```python
from build123d import *

# Parameters (mm, degrees)
SKETCH_1_R          = 5.05
SKETCH_1_R_2        = 13
EXTRUDE_1_DEPTH     = 12
FILLET_1_R          = 3
CUT_EXTRUDE_3_DEPTH = 277.39464539
FILLET_2_R          = 3
EXTRUDE_START       = -12
SKETCH_5_R          = 40
SKETCH_5_R_2        = 5.05
EXTRUDE_2_DEPTH     = 12
FILLET_3_R          = 6
EXTRUDE_3_DEPTH     = 12
FILLET_4_R          = 3
SKETCH_8_R          = 32
CUT_EXTRUDE_5_DEPTH = 279.152835686


with BuildPart() as part:
    # 草图1 → 凸台-拉伸1 (new body)
    with BuildSketch(Plane(origin=(0, 0, 0), x_dir=(1, 0, 0), z_dir=(0, 1, 0))):
        with BuildLine():
            Line((-17.992942616, -0.504), (-24.990198078, 249.3))
            ThreePointArc((-24.990198078, 249.3), (0, 275), (24.990198078, 249.3))
            Line((24.990198078, 249.3), (17.992942616, -0.504))
            ThreePointArc((17.992942616, -0.504), (0, -18), (-17.992942616, -0.504))
        make_face()
        with Locations(Location((0, 0, 0), (0, 0, 270))):
            Circle(SKETCH_1_R, mode=Mode.SUBTRACT)
        with Locations(Location((0, 250, 0), (0, 0, 270))):
            Circle(SKETCH_1_R_2, mode=Mode.SUBTRACT)
        Polygon((-16.444447487, 158.5), (-17.704941698, 203.5), (11.028871219, 137.174942267), align=None, mode=Mode.SUBTRACT)
        Polygon((15.954255294, 141), (18.475243716, 231), (-12, 219.5), align=None, mode=Mode.SUBTRACT)
    extrude(amount=EXTRUDE_1_DEPTH)

    # 圆角1
    fillet_1_edges = [part.edges().sort_by_distance(p)[0] for p in [
        (-16.444447487, 6, -158.5),
        (11.028871219, 6, -137.174942267),
        (-17.704941698, 6, -203.5),
        (18.475243716, 6, -231),
        (-12, 6, -219.5),
        (15.954255294, 6, -141),
    ]]
    fillet(fillet_1_edges, radius=FILLET_1_R)

    # 草图4 → 切除-拉伸3 (cut, through all)
    with BuildSketch(Plane(origin=(0, 12, 0), x_dir=(1, 0, 0), z_dir=(0, 1, 0))):
        Polygon((-13.050343026, 144.472367448), (12.494927596, 124.643879429), (9.742058902, 26.365688077), (-10.175105816, 41.825585442), align=None)
    extrude(amount=-CUT_EXTRUDE_3_DEPTH, mode=Mode.SUBTRACT)

    # 圆角2
    fillet_2_edges = [part.edges().sort_by_distance(p)[0] for p in [
        (-10.175105816, 6, -41.825585442),
        (-13.050343026, 6, -144.472367448),
        (9.742058902, 6, -26.365688077),
    ]]
    fillet(fillet_2_edges, radius=FILLET_2_R)

    # 草图5 → 凸台-拉伸2 (add)
    with BuildSketch(Plane(origin=(0, 12, 0), x_dir=(1, 0, 0), z_dir=(0, 1, 0)).offset(EXTRUDE_START)):
        Circle(SKETCH_5_R)
        with Locations(Location((0, 0, 0), (0, 0, 270))):
            Circle(SKETCH_5_R_2, mode=Mode.SUBTRACT)
    extrude(amount=EXTRUDE_2_DEPTH)

    # 圆角3
    fillet_3_edges = [part.edges().sort_by_distance(p)[0] for p in [
        (18.993134598, 6, -35.203136766),
        (-18.993134598, 6, -35.203136766),
    ]]
    fillet(fillet_3_edges, radius=FILLET_3_R)

    # 草图6 → 凸台-拉伸3 (add)
    with BuildSketch(Plane(origin=(0, 12, 0), x_dir=(1, 0, 0), z_dir=(0, 1, 0))):
        Polygon((9.60137553, 125.435937788), (-13.068657882, 42.617643801), (-7.609801347, 39.834371112), (-7.28155375, 41.033527083), (15.388479662, 123.85182107), (9.929623127, 126.635093759), align=None)
    extrude(amount=-EXTRUDE_3_DEPTH)

    # 圆角4
    # the kernel refuses this fillet: 3 mm, written as the material it adds along each edge
    with BuildSketch(Plane(origin=(12.14036175, 0, -111.985778385), x_dir=(-0.028000000000000382, 0, 0.9996079231378672), z_dir=(0, 1, 0))) as fillet_4_piece_1:
        with BuildLine():
            CenterArc((FILLET_4_R * 8.32187878655, -FILLET_4_R), FILLET_4_R, 90, 166.295794849)
            Line((FILLET_4_R * 8.08496933551, -FILLET_4_R * 1.97153173495), (FILLET_4_R * 8.08023114649, -FILLET_4_R * 1.99096236965))
            Line((FILLET_4_R * 8.08023114649, -FILLET_4_R * 1.99096236965), (-FILLET_4_R * 0.0047381890208, -FILLET_4_R * 0.0194306346989))
            Line((-FILLET_4_R * 0.0047381890208, -FILLET_4_R * 0.0194306346989), (0, FILLET_4_R * 0.02))
            Line((0, FILLET_4_R * 0.02), (FILLET_4_R * 8.32187878655, FILLET_4_R * 0.02))
            Line((FILLET_4_R * 8.32187878655, FILLET_4_R * 0.02), (FILLET_4_R * 8.32187878655, 0))
        make_face()
    extrude(amount=12)
    with BuildSketch(Plane(origin=(-10.463842583, 0, -52.133569747), x_dir=(-0.02799999999999904, 0, -0.9996079231378672), z_dir=(0, 1, 0))) as fillet_4_piece_2:
        with BuildLine():
            CenterArc((FILLET_4_R * 6.72600834912, -FILLET_4_R), FILLET_4_R, 90, 163.086811796)
            Line((FILLET_4_R * 6.43508592619, -FILLET_4_R * 1.95674664558), (FILLET_4_R * 6.42926747773, -FILLET_4_R * 1.9758815785))
            Line((FILLET_4_R * 6.42926747773, -FILLET_4_R * 1.9758815785), (-FILLET_4_R * 0.00581844845863, -FILLET_4_R * 0.0191349329117))
            Line((-FILLET_4_R * 0.00581844845863, -FILLET_4_R * 0.0191349329117), (0, FILLET_4_R * 0.02))
            Line((0, FILLET_4_R * 0.02), (FILLET_4_R * 6.72600834912, FILLET_4_R * 0.02))
            Line((FILLET_4_R * 6.72600834912, FILLET_4_R * 0.02), (FILLET_4_R * 6.72600834912, 0))
        make_face()
    extrude(amount=12)
    with BuildSketch(Plane(origin=(9.929623127, 12, -126.635093759), x_dir=(-0.7899521186549702, 0, -0.6131685333026506), z_dir=(0, -1, 0))) as fillet_4_piece_3:
        with BuildLine():
            CenterArc((FILLET_4_R * 0.668049057951, -FILLET_4_R), FILLET_4_R, 90, 67.489733811)
            Line((-FILLET_4_R * 0.255761890972, -FILLET_4_R * 0.617151034153), (-FILLET_4_R * 0.27423810995, -FILLET_4_R * 0.609494054836))
            Line((-FILLET_4_R * 0.27423810995, -FILLET_4_R * 0.609494054836), (-FILLET_4_R * 0.013360981159, FILLET_4_R * 0.02))
            Line((-FILLET_4_R * 0.013360981159, FILLET_4_R * 0.02), (FILLET_4_R * 0.668049057951, FILLET_4_R * 0.02))
            Line((FILLET_4_R * 0.668049057951, FILLET_4_R * 0.02), (FILLET_4_R * 0.668049057951, 0))
        make_face()
    extrude(amount=12)
    with BuildSketch(Plane(origin=(-7.609801347, 12, -39.834371112), x_dir=(0.789952118654971, 0, 0.6131685333026496), z_dir=(0, -1, 0))) as fillet_4_piece_4:
        with BuildLine():
            CenterArc((2.149138752, -2.650136686), FILLET_4_R, 117.947316923, 39.542416888)
            Line((-0.622294094, -1.501589789), (-0.677722751, -1.478618851))
            Line((-0.677722751, -1.478618851), (-0.055428657, 0.022970938))
            Line((-0.055428657, 0.022970938), (0, 0.06))
            ThreePointArc((0, 0.06), (0.371580126, 0.06), (0.715040682, 0.053002734))
            Line((0.715040682, 0.053002734), (0.743160252, 0))
        make_face()
    extrude(amount=12)

    # 草图8 → 切除-拉伸5 (cut, through all)
    with BuildSketch(Plane(origin=(0, 12, 0), x_dir=(1, 0, 0), z_dir=(0, 1, 0))):
        with Locations(Location((0, 0, 0), (0, 0, 270))):
            Circle(SKETCH_8_R)
    extrude(amount=-CUT_EXTRUDE_5_DEPTH, mode=Mode.SUBTRACT)


solid = part.part
```
Can you work these out from the model? Positions are in its coordinate system, mm. A direction names the side the tool comes from. Coordinates: 2 decimals unless noted, no trailing zeros. Loops run counter-clockwise (first coordinate to the right, second up) from the corner with the lowest first, then second, coordinate; pieces in that order, holes last. Notation, with made-up numbers: (67, 24) -> (120, 24) arc R21 ccw to (120, 60) -> close; hole circle Ø3 at (31.25, 44). An arc over 180 degrees is marked (long way). Put each result on its own line as item: value. Start each with the question number.
Q1. I want a section at B-B (y = 7.5). Count the separate pieces of the cut face and the enclosed holes in it, plus the area to 3 significant figures.
Q2. For faces 1 (the face through (2.688, 5.916, -225.043)), 2 (the face through (19.796, 5.916, -35.731)), which set-ups out of +Z, -Z, +X, -X, +Y, -Y let a thin tool reach every point of the face, with its end or its side?
Q3. I want a section at A-A (z = 0). Write out the boundary of the cut face in (x, y).
Q4. I'm going to push flat-ended pins straight in: P1, Ø4, axis at y = 3, z = -163.5, coming from the +X side; P2, Ø3, axis at x = -30.5, y = 7.5, coming from the -Z side; P3, Ø2, axis at x = 7.5, z = -111, coming from the -Y side; P4, Ø5, axis at x = 24, y = 3, coming from the -Z side. Where does each tip first touch, or does it pass through?
Q5. If I drill on line 1 (X direction, y = 7, z = 0); line 2 (X direction, y = 11.25, z = -185.5); line 3 (X direction, y = 6, z = -250), over which ranges is the centre line in solid material (lowest first)? Write a range as [from, to].
Q6. Thinking about a two-plate mould opening in Z: for faces 3 (the face through (8, 0, -109)), 4 (the face through (-19.796, 5.916, -35.731)), which applies, pulls with the +Z half, pulls with the -Z half, needs draft (parallel to the pull), parting line crosses it, or undercut?
Q7. I want a section at C-C (z = -101). Write out the boundary of the cut face in (x, y), plus the area to 3 significant figures.
Taken from the geometry:
1. separate pieces: 1
1. enclosed holes: 6
1. area: 8,170 mm2
2. face 1: +Y, -Y
2. face 2: +X, +Y, -Y
3. outline: (-40, 0) -> (-32, 0) -> (-32, 12) -> (-40, 12) -> close; (32, 0) -> (40, 0) -> (40, 12) -> (32, 12) -> close
4. P1: stops at x = 22.64
4. P2: stops at z = -27.55
4. P3: stops at y = 0
4. P4: stops at z = -262.76
5. line 1: x = [-40, -32], [32, 40]
5. line 2: x = [-23.2, -17.2], [-9.91, 0.11], [17.2, 23.2]
5. line 3: x = [-25, -13], [13, 25]
6. face 3: needs draft
6. face 4: undercut
7. outline: (-20.84, 0) -> (-11.83, 0) -> (-11.83, 12) -> (-20.84, 12) -> close; (2.91, 0) -> (20.84, 0) -> (20.84, 12) -> (2.91, 12) -> close
7. area: 323 mm2
